Verification items for the finished model (mm, model axes). A direction names the side the tool comes from. Coordinates: 2 decimals unless noted, no trailing zeros. Loops run counter-clockwise (first coordinate to the right, second up) from the corner with the lowest first, then second, coordinate; pieces in that order, holes last. Notation, with made-up numbers: (86, 57.25) - (122, 57.25) arc R22 ccw to (122, 92.25) - close; hole circle Ø5 at (-37.75, 87.25). An arc over 180 degrees is marked (long way). One line per item, written item: value. Start each with the question number.
(1) Section check B-B (y = 13). Count the separate pieces of the cut face and the enclosed holes in it, plus the area to 3 significant figures.
(2) Draft check along X on faces 4 (the face through (-101.767, 9.86, -1.341)), 5 (the face through (59.185, 9.86, -82.511)), 6 (the face through (-101, 10, -10)). Enter one of: +X half, -X half, draft (parallel to the pull), parting line (faces both ways), or undercut.
(3) Gauge pin test, flat ends, axial feed: P1, Ø9.5, axis at x = 72.5, z = 71, coming from the -Y side; P2, Ø1.5, axis at y = 43.5, z = 7.5, coming from the +X side; P3, Ø2, axis at x = 0, z = 26.5, coming from the +Y side; P4, Ø4, axis at x = 26.5, z = 0, coming from the +Y side. Record the tip position at first contact, or that the pin passes through.
(4) Thickness scan on probe 1 along Z at (x, y) = (0, 76); probe 2 along X at (y, z) = (114.5, 70.71); probe 3 along X at (y, z) = (114, 70). Record the ranges inside material, lowest first. Write a range as [from, to].
(5) Set-up check for faces 1 (the face through (-63.714, 118.225, -63.564)), 2 (the face through (52, 20, 95)), 3 (the face through (27, 40, -45)): record each of +Z, -Z, +X, -X, +Y, -Y from which the full face is reachable in a straight line by a thin tool's end or side.
(6) Section check D-D (y = 43). Record the boundary of the cut face in (x, z).
(7) Section check C-C (y = 102). Record the boundary of the cut face in (x, z).
(8) Section check A-A (y = 79). Record the boundary of the cut face in (x, z).
```python
from build123d import *

# Parameters (mm, degrees)
ESBO_O4_R                = 10
RESSALTO_EXTRUS_O1_DEPTH = 35
RESSALTO_EXTRUS_O2_DEPTH = 20
ESBO_O8_R                = 3.5
CORTE_EXTRUS_O2_DEPTH    = 20
PADR_OCIRCULAR1_COUNT    = 6
ESBO_O6_R                = 3.5
CORTE_EXTRUS_O1_DEPTH    = 15
ESBO_O9_R                = 1.25
CORTE_EXTRUS_O3_DEPTH    = 6


with BuildPart() as part:
    # Esboço3 → Revolução2 (revolve)
    with BuildSketch(Plane.XY):
        with BuildLine():
            Line((97.5, 120), (97.5, 11.304491341))
            Line((97.5, 11.304491341), (97.5, 0))
            Line((97.5, 0), (82.842408243, 0))
            Line((82.842408243, 0), (60.342408243, 0))
            Line((60.342408243, 0), (60.342408243, 40))
            Line((60.342408243, 40), (52, 40))
            Line((52, 40), (44, 48))
            Line((44, 48), (31, 48))
            Line((31, 48), (31, 50.75))
            Line((31, 50.75), (22.6, 50.75))
            Line((22.6, 50.75), (22.6, 54.05))
            Line((22.6, 54.05), (19.3, 54.05))
            Line((19.3, 54.05), (19.3, 54.75))
            Line((19.3, 54.75), (15.3, 54.75))
            Line((15.3, 54.75), (15.3, 58.1))
            Line((15.3, 58.1), (19.3, 58.1))
            Line((19.3, 58.1), (19.3, 58.25))
            Line((19.3, 58.25), (27.626549127, 66.16))
            Line((27.626549127, 66.16), (31.3, 66.16))
            Line((31.3, 66.16), (31.3, 84.16))
            Line((31.3, 84.16), (32.3, 85.16))
            Line((32.3, 85.16), (38.8, 85.16))
            Line((38.8, 85.16), (38.8, 67.1))
            Line((38.8, 67.1), (55.5, 50.4))
            Line((55.5, 50.4), (83.5, 50.4))
            ThreePointArc((83.5, 50.4), (86.328427125, 51.571572875), (87.5, 54.4))
            Line((87.5, 54.4), (87.5, 116.4))
            Line((87.5, 116.4), (93, 116.4))
            Line((93, 116.4), (93, 120))
            Line((93, 120), (97.5, 120))
        make_face()
    revolve(axis=Axis((0, -3.631214097, 0), (0, 1, 0)))

    # Esboço4 → Ressalto-extrusão1 (add)
    with BuildSketch(Plane(origin=(0, 120, 0), x_dir=(1, 0, 0), z_dir=(0, 1, 0))):
        with Locations((70.71, 70.71)):
            Circle(ESBO_O4_R)
        with Locations((70.71, -70.71)):
            Circle(ESBO_O4_R)
        with Locations((-70.71, -70.71)):
            Circle(ESBO_O4_R)
        with Locations((-70.71, 70.71)):
            Circle(ESBO_O4_R)
    extrude(amount=-RESSALTO_EXTRUS_O1_DEPTH)

    # Esboço5 → Ressalto-extrusão2 (add)
    with BuildSketch(Plane.XZ):
        with BuildLine():
            Line((-105, -10), (-96.985823706, -10))
            Line((-96.985823706, -10), (-96.985823706, 10))
            Line((-96.985823706, 10), (-105, 10))
            ThreePointArc((-105, 10), (-115, 0), (-105, -10))
        make_face()
    ressalto_extrus_o2 = extrude(amount=-RESSALTO_EXTRUS_O2_DEPTH)

    # Esboço8 → Corte-extrusão2 (cut)
    with BuildSketch(Plane.XZ):
        with Locations((-105, 0)):
            Circle(ESBO_O8_R)
    corte_extrus_o2 = extrude(amount=-CORTE_EXTRUS_O2_DEPTH, mode=Mode.SUBTRACT)

    # PadrãoCircular1: Ressalto-extrusão2, Corte-extrusão2 ×6 about axis
    padr_ocircular1_axis = Axis((0, 0, 0), (0, 1, 0))
    for i in range(1, PADR_OCIRCULAR1_COUNT):
        add(ressalto_extrus_o2.rotate(padr_ocircular1_axis, i * 360 / PADR_OCIRCULAR1_COUNT))
        add(corte_extrus_o2.rotate(padr_ocircular1_axis, i * 360 / PADR_OCIRCULAR1_COUNT), mode=Mode.SUBTRACT)

    # Esboço6 → Corte-extrusão1 (cut)
    with BuildSketch(Plane(origin=(0, 120, 0), x_dir=(1, 0, 0), z_dir=(0, 1, 0))):
        with Locations((-70.71, -70.71)):
            Circle(ESBO_O6_R)
        with Locations((70.71, -70.71)):
            Circle(ESBO_O6_R)
        with Locations((70.71, 70.71)):
            Circle(ESBO_O6_R)
        with Locations((-70.71, 70.71)):
            Circle(ESBO_O6_R)
    extrude(amount=-CORTE_EXTRUS_O1_DEPTH, mode=Mode.SUBTRACT)

    # Esboço9 → Corte-extrusão3 (cut)
    with BuildSketch(Plane.XZ.offset(-50.75)):
        with Locations((0, 26.5)):
            Circle(ESBO_O9_R)
        with Locations((26.5, 0)):
            Circle(ESBO_O9_R)
        with Locations((0, -26.5)):
            Circle(ESBO_O9_R)
        with Locations((-26.5, 0)):
            Circle(ESBO_O9_R)
    extrude(amount=-CORTE_EXTRUS_O3_DEPTH, mode=Mode.SUBTRACT)


solid = part.part
```
Responses:
1. separate pieces: 1
1. enclosed holes: 7
1. area: 20,100 mm²
2. face 4: undercut
2. face 5: +X half
2. face 6: draft
3. P1: stops at y = 0
3. P2: stops at x = 97.27
3. P3: stops at y = 66.04
3. P4: stops at y = 66.16
4. probe 1: z = [-97.5, -87.5], [-38.8, -31.3], [31.3, 38.8], [87.5, 97.5]
4. probe 2: x = [-80.71, -74.21], [-67.21, -51.54], [51.54, 67.21], [74.21, 80.71]
4. probe 3: x = [-80.68, -74.14], [-67.28, -52.5], [52.5, 67.28], [74.14, 80.68]
5. face 1: +Y
5. face 2: +Z, +X, +Y
5. face 3: -Y
6. outline: circle Ø195 at (0, 0); hole circle Ø98 at (0, 0)
7. outline: (-75.36, -61.86) arc R10 ccw (long way) to (-61.86, -75.36) arc R97.5 ccw to (61.86, -75.36) arc R10 ccw (long way) to (75.36, -61.86) arc R97.5 ccw to (75.36, 61.86) arc R10 ccw (long way) to (61.86, 75.36) arc R97.5 ccw to (-61.86, 75.36) arc R10 ccw (long way) to (-75.36, 61.86) arc R97.5 ccw to start; hole circle Ø175 at (0, 0)
8. outline: circle Ø195 at (0, 0); circle Ø77.6 at (0, 0); hole circle Ø175 at (0, 0); hole circle Ø62.6 at (0, 0)
